from build123d import *

# Parameters (mm, degrees)
SKETCH_1_W          = 3
SKETCH_1_H          = 4
SKETCH_2_R          = 3.5
CUT_EXTRUDE_1_DEPTH = 0.2
SKETCH_3_R          = 5.5
SKETCH_3_R_2        = 4
CUT_EXTRUDE_2_DEPTH = 0.2


with BuildPart() as part:
    # Эскиз1 → Повернуть1 (revolve)
    with BuildSketch(Plane(origin=(0, 0, 0), x_dir=(1, 0, 0), z_dir=(0, 1, 0))):
        with Locations((-4.5, 2)):
            Rectangle(SKETCH_1_W, SKETCH_1_H)
    revolve(axis=Axis((0, 0, 0), (0, 0, -1)))

    # Эскиз2 → Вырез-Вытянуть1 (cut)
    with BuildSketch(Plane.XY):
        Circle(SKETCH_2_R)
    cut_extrude_1 = extrude(amount=-CUT_EXTRUDE_1_DEPTH, mode=Mode.SUBTRACT)

    # Эскиз3 → Вырез-Вытянуть2 (cut)
    with BuildSketch(Plane.XY):
        Circle(SKETCH_3_R)
        Circle(SKETCH_3_R_2, mode=Mode.SUBTRACT)
    cut_extrude_2 = extrude(amount=-CUT_EXTRUDE_2_DEPTH, mode=Mode.SUBTRACT)

    # Зеркальное отражение1: Вырез-Вытянуть1, Вырез-Вытянуть2 across plane
    add(cut_extrude_1.mirror(Plane.XY.offset(-2)), mode=Mode.SUBTRACT)
    add(cut_extrude_2.mirror(Plane.XY.offset(-2)), mode=Mode.SUBTRACT)


solid = part.part
Geometry check sheet. Reference: the model listing, model coordinates, mm. A direction names the side the tool comes from. Give positions to 0.01 mm unless a question says otherwise; leave off trailing zeros. Loops run counter-clockwise (first coordinate to the right, second up) from the corner with the lowest first, then second, coordinate; pieces in that order, holes last. Notation, with made-up numbers: M 76.25,-15.75 L 122.25,-15.75 A18 ccw 122.25,17.25 Z; hole C 32.25,11 d10. An arc over 180 degrees is marked long. Answer as a JSON object with one key per item and string values. Group by question number.
Item 1: Gauge pin test, flat ends, axial feed: pin 1 (1.5 mm diameter, centred on y = 4.5, z = -2, fed in from +X); pin 2 (5 mm diameter, centred on x = -3.5, y = -3, fed in from +Z); pin 3 (1.5 mm diameter, centred on y = 1.5, z = -1.5, fed in from -X); pin 4 (2 mm diameter, centred on y = 2.5, z = -0.5, fed in from -X). Record the tip position at first contact, or that the pin passes through.
Item 2: Mould release check, pull along X, two halves, no side actions. Record for faces 4 (the flat face through (3, 1, -3.8)), 5 (the flat face through (-3, -5, 0)), 6 (the cylindrical face through (6, 0, -2)): pulls with the +X half, pulls with the -X half, needs draft (parallel to the pull), parting line crosses it, or undercut.
Item 3: Sectioned sample at D-D on x = -4.5. Record the boundary of the cut face in (y, z), plus the area to 3 significant figures.
Item 4: Access from +Z, -Z, +X, -X, +Y, -Y to the whole of each face (thin tool, end or side, straight path). Record for faces 1 (the flat face through (-4, -2, -3.8)), 2 (the flat face through (-4, -2, -0.2)), 3 (the cylindrical face through (3, 0, -2)).
Item 5: Sectioned sample at C-C on z = -2.4. Record the boundary of the cut face in (x, y).
Item 6: Material ranges on L1, parallel to Y at x = 0, z = -0.1; L2, parallel to Y at x = 0, z = -0.95; L3, parallel to Z at x = 1, y = 5.25, recorded low to high.
Findings below:
{
 "1": {"pin 1": "x = 4.68", "pin 2": "z = 0", "pin 3": "x = -5.95", "pin 4": "x = -5.81"},
 "2": {"face 4": "undercut", "face 5": "needs draft", "face 6": "parting line crosses it"},
 "3": {"outline": "M -3.97,-4 L -3.16,-4 L -3.16,-3.8 L 3.16,-3.8 L 3.16,-4 L 3.97,-4 L 3.97,0 L 3.16,0 L 3.16,-0.2 L -3.16,-0.2 L -3.16,0 L -3.97,0 Z", "area": "29.2 mm2"},
 "4": {"face 1": "-Z", "face 2": "+Z", "face 3": "+Z, -Z"},
 "5": {"outline": "C 0,0 d12; hole C 0,0 d6"},
 "6": {"L1": "-6 to -5.5, -4 to -3.5, 3.5 to 4, 5.5 to 6", "L2": "-6 to -3, 3 to 6", "L3": "-3.8 to -0.2"}
}
